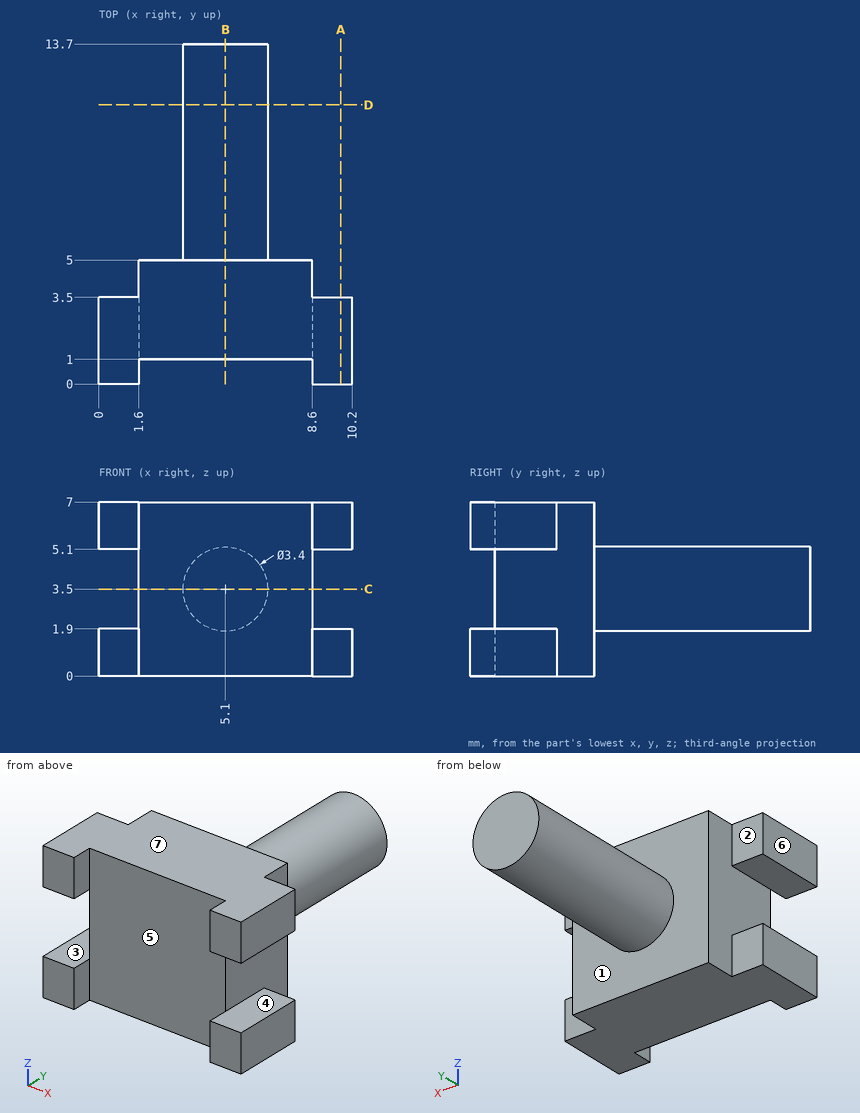
The drawing under review shows one solid part. Ordinate dimensions are in mm from its lowest x, y, z. A direction names the side the tool comes from. Round coordinates to 2 decimals unless told otherwise and drop trailing zeros. Write each loop counter-clockwise with the first axis right and the second up, starting at its lowest first coordinate (ties: lowest second). Pieces come first, ordered by that corner, then holes. Notation, with made-up numbers: (-38, 67.25) - (-3, 67.25) arc R15 cw to (-3, 90.25) - close; hole circle Ø2 at (12.5, 30.25). An arc over 180 degrees is marked (long way). Write each question's results on one line, items separated by ' | '.
Item 1: For pin 1 (1.3 mm diameter, centred on x = 9.5, z = 0.5, fed in from +Y); pin 2 (1.3 mm diameter, centred on x = 1, z = 1, fed in from +Y); pin 3 (1.2 mm diameter, centred on y = 4, z = 3, fed in from -X); pin 4 (1.5 mm diameter, centred on x = 2, y = 9.5, fed in from +Z), all flat-tipped, find the tip position at first contact; note any pin that passes through.
Calculated:
pin 1: stops at y = 3.5 | pin 2: stops at y = 5 | pin 3: stops at x = 1.6 | pin 4: passes through
Item 2: For the marked faces 1, 2, 3 and 4, list the 3-axis set-ups (+Z, -Z, +X, -X, +Y, -Y) from which the entire face can be reached by the end or side of a thin tool; tool diameter is ignored.
Calculated:
face 1: +Y | face 2: +Z, -Z, -X, +Y | face 3: -X, +Y, -Y | face 4: +X, +Y, -Y
Item 3: Take a section at B-B on x = 5.1. State the section outline as (y, z) points, then the cut area to 3 significant figures.
Calculated:
outline: (1, 0) - (5, 0) - (5, 1.8) - (13.7, 1.8) - (13.7, 5.2) - (5, 5.2) - (5, 7) - (1, 7) - close | area: 57.6 mm^2
Item 4: Take a section at D-D on y = 11.25. State the section outline as (x, z) points, then the cut area to 3 significant figures.
Calculated:
outline: circle Ø3.4 at (5.1, 3.5) | area: 9.08 mm^2
Item 5: Take a section at A-A on x = 9.75. State the section outline as (y, z) points.
Calculated:
outline: (0, 0) - (3.5, 0) - (3.5, 1.9) - (0, 1.9) - close; (0, 5.1) - (3.5, 5.1) - (3.5, 7) - (0, 7) - close
Item 6: Take a section at C-C on z = 3.5. State the section outline as (x, y) points, then the cut area to 3 significant figures.
Calculated:
outline: (1.6, 1) - (8.6, 1) - (8.6, 5) - (6.8, 5) - (6.8, 13.7) - (3.4, 13.7) - (3.4, 5) - (1.6, 5) - close | area: 57.6 mm^2
Item 7: To check wall thickness, follow line 1 along Y through (x, z) = (1.75, 5); line 2 along Z through (x, y) = (5, 9.25); line 3 along X through (y, z) = (3.75, 4.5). State the ranges of each line that lie inside material, in increasing order. Write a range as from..to.
Calculated:
line 1: y = 1..5 | line 2: z = 1.8..5.2 | line 3: x = 1.6..8.6
Item 8: Draft analysis for pull direction X (two halves, no side actions). For the marked faces 5, 6 and 7, state which applies: pulls with the +X half, pulls with the -X half, needs draft (parallel to the pull), parting line crosses it, or undercut.
Calculated:
face 5: undercut | face 6: pulls with the -X half | face 7: needs draft
